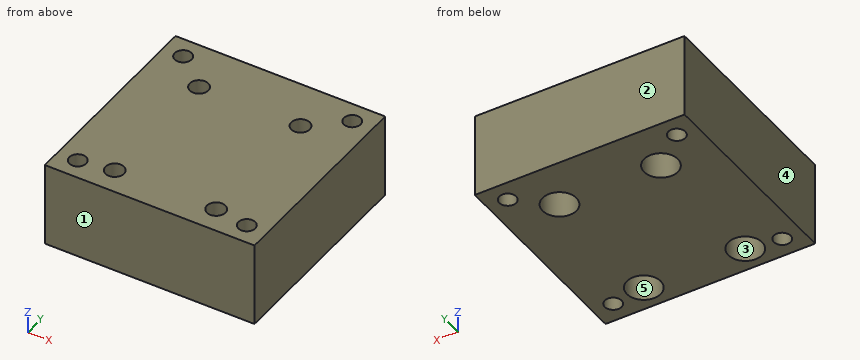
from build123d import *

# Parameters (mm, degrees)
SKETCH_1_W                   = 62
SKETCH_1_H                   = 62
EXTRUDE_1_DEPTH              = 25
HOLE_WIZARD_M6_1_D           = 5
HOLE_WIZARD_M5_1_D           = 5.5
HOLE_WIZARD_M5_1_CBORE_D     = 10
HOLE_WIZARD_M5_1_CBORE_DEPTH = 20


with BuildPart() as part:
    # 草图1 → 凸台-拉伸1 (new body)
    with BuildSketch(Plane.XY):
        Rectangle(SKETCH_1_W, SKETCH_1_H)
    extrude(amount=EXTRUDE_1_DEPTH)

    # M6 螺纹孔1 (through all)
    with Locations(Plane(origin=(25, 25, 0), x_dir=(-1, 0, 0), z_dir=(0, 0, -1))):
        with Locations((0, 0), (50, 0), (0, -50), (50, -50)):
            Hole(HOLE_WIZARD_M6_1_D / 2)

    # M5 六角凹头螺钉的柱形沉头孔1 (through all)
    with Locations(Plane(origin=(15, 16.5, 0), x_dir=(-1, 0, 0), z_dir=(0, 0, -1))):
        with Locations((0, 0), (30, 0), (30, -40), (0, -40)):
            CounterBoreHole(HOLE_WIZARD_M5_1_D / 2, HOLE_WIZARD_M5_1_CBORE_D / 2, HOLE_WIZARD_M5_1_CBORE_DEPTH)


solid = part.part
Geometry: final body of the model. Coordinates: model frame, mm. Face numbers are marked on the shaded views. A direction names the side the tool comes from. Coordinates: 2 decimals unless noted, no trailing zeros. Order: outer loops, then holes, each group sorted by start corner. A loop starts at its lowest first (then second) coordinate and runs counter-clockwise, first axis right, second up. Notation, with made-up numbers: (-26.5, 69) - (5.5, 69) arc R12 cw to (5.5, 91) - close; hole circle Ø7 at (-14, 2). An arc over 180 degrees is marked (long way). Use one line per item in the form item = value.
1) Section B-B (y = -23.5). Return loops of the section in (x, z), then the cut area to 3 significant figures.
Solutions:
outline = (-31, 0) - (-27, 0) - (-27, 25) - (-31, 25) - close; (-23, 0) - (-20, 0) - (-20, 20) - (-17.75, 20) - (-17.75, 25) - (-23, 25) - close; (-12.25, 20) - (-10, 20) - (-10, 0) - (10, 0) - (10, 20) - (12.25, 20) - (12.25, 25) - (-12.25, 25) - close; (17.75, 20) - (20, 20) - (20, 0) - (23, 0) - (23, 25) - (17.75, 25) - close; (27, 0) - (31, 0) - (31, 25) - (27, 25) - close
area = 895 mm^2
2) Set-up query: the marked faces 4 and 5. Return all of +Z, -Z, +X, -X, +Y, -Y with unobstructed straight access to the full face (end or side cutting, diameter ignored); none if empty.
Solutions:
face_4 = +Z, -Z, -X, +Y, -Y
face_5 = -Z
3) Section A-A (x = -25). Return loops of the section in (y, z).
Solutions:
outline = (-31, 0) - (-27.5, 0) - (-27.5, 25) - (-31, 25) - close; (-22.5, 0) - (22.5, 0) - (22.5, 25) - (-22.5, 25) - close; (27.5, 0) - (31, 0) - (31, 25) - (27.5, 25) - close
4) Section C-C (z = 18.25). State how many separate pieces and enclosed holes the cut face has, then the cut area to 3 significant figures.
Solutions:
separate_pieces = 1
enclosed_holes = 8
area = 3,450 mm^2
5) Pin query (flat end, axial travel): pin 1 (3 mm diameter, centred on x = -13.5, y = -24, fed in from -Z). Return the tip coordinate at first contact, or that it passes through.
Solutions:
pin_1 = 20
6) Section D-D (y = 16.5). Return loops of the section in (x, z), then the cut area to 4 significant figures.
Solutions:
outline = (-31, 0) - (-20, 0) - (-20, 20) - (-17.75, 20) - (-17.75, 25) - (-31, 25) - close; (-12.25, 20) - (-10, 20) - (-10, 0) - (10, 0) - (10, 20) - (12.25, 20) - (12.25, 25) - (-12.25, 25) - close; (17.75, 20) - (20, 20) - (20, 0) - (31, 0) - (31, 25) - (17.75, 25) - close
area = 1,095 mm^2
7) Mould query, pull axis Y, two halves, no side actions, for the marked faces 1, 2 and 3. Classes: +Y half, -Y half, draft (parallel to the pull), parting line (faces both ways), or undercut.
Solutions:
face_1 = -Y half
face_2 = +Y half
face_3 = undercut
8) Ray query, L1, parallel to Y at x = -15, z = 15.5; L2, parallel to Y at x = -25, z = 16.5; L3, parallel to X at y = 21, z = 18. Return the intervals inside material, ascending.
Solutions:
L1 = -31 to -28.5, -18.5 to 11.5, 21.5 to 31
L2 = -31 to -27.5, -22.5 to 22.5, 27.5 to 31
L3 = -31 to -17.18, -12.82 to 12.82, 17.18 to 31
